from build123d import *

# Parameters (mm, degrees)
EXTRUDE_1_DEPTH = 2
SKETCH_2_R      = 4.1
EXTRUDE_2_DEPTH = 15


with BuildPart() as part:
    # 草图1 → 凸台-拉伸1 (new body)
    with BuildSketch(Plane.XY):
        Polygon((-12.668616293, 22.288540635), (-0.168616293, 22.288540635), (-0.168616293, 19.288540635), (14.831383707, 19.288540635), (14.831383707, 22.288540635), (27.331383707, 22.288540635), (27.331383707, -2.711459365), (-12.668616293, -2.711459365), align=None)
        with BuildLine():
            Line((-7.668616293, 0.038540635), (22.331383707, 0.038540635))
            ThreePointArc((22.331383707, 0.038540635), (23.081383707, -0.711459365), (22.331383707, -1.461459365))
            Line((22.331383707, -1.461459365), (-7.668616293, -1.461459365))
            ThreePointArc((-7.668616293, -1.461459365), (-8.418616293, -0.711459365), (-7.668616293, 0.038540635))
        make_face(mode=Mode.SUBTRACT)
    extrude(amount=EXTRUDE_1_DEPTH)

    # 草图2 → 凸台-拉伸2 (add)
    with BuildSketch(Plane(origin=(0, 19.288540635, 0), x_dir=(1, 0, 0), z_dir=(0, 1, 0))):
        with BuildLine():
            Line((4.831383707, 2.381058819), (4.831383707, 0))
            Line((4.831383707, 0), (9.831383707, 0))
            Line((9.831383707, 0), (9.831383707, 2.399323324))
            ThreePointArc((9.831383707, 2.399323324), (7.288775956, 14.054276854), (4.831383707, 2.381058819))
        make_face()
        with Locations((7.311058504, 7.954317551)):
            Circle(SKETCH_2_R, mode=Mode.SUBTRACT)
    extrude(amount=-EXTRUDE_2_DEPTH)


solid = part.part
CAD build for the part. Positions are in the model's coordinates, mm. A direction names the side the tool comes from. Round coordinates to 2 decimals unless told otherwise and drop trailing zeros. Write each loop counter-clockwise with the first axis right and the second up, starting at its lowest first coordinate (ties: lowest second). Pieces come first, ordered by that corner, then holes. Notation, with made-up numbers: M 41,-18.75 L 61,-18.75 A31 cw 61,20.25 Z; hole C 78,-20 d5. An arc over 180 degrees is marked long. Use a Markdown table: item, result. Add a question column.
1. Pull direction Z, two halves, no side cores. Call faces 1 (the face through (3, 4.289, -7)), 2 (the face through (6.78, 11.89, -12.02)), 3 (the face through (8, 10, 2)): released by +Z, released by -Z, zero draft, split by the parting line, or undercut.
2. Drill centre lines: probe 1 along Z at (x, y) = (-6, 19.25); probe 2 along Y at (x, z) = (9.5, -1.75); probe 3 along Y at (x, z) = (-6, 1). Where is each one in solid material? Low to high.
3. Flat gauge pins, fed straight in: P1, Ø4.5, axis at x = 8.5, z = -5, coming from the +Y side; P2, Ø1.9, axis at y = 10.5, z = -1, coming from the +X side; P3, Ø0.7, axis at y = 14, z = -1, coming from the -X side. Where does each tip first touch, or does it go through?
4. Slice it at B-B on z = -5.75. Give the cut face in (x, y), then the cut area to 3 significant figures.
5. Slice it at D-D on x = 6. Give the cut face in (y, z).
6. Slice it at A-A on x = 14. Give the cut face in (y, z).
7. 3-axis set-ups, long thin cutter, end or side, ignore diameter. For faces 4 (the face through (-8.42, -0.73, 0.99)), 5 (the face through (-0.169, 21, 1)), 6 (the face through (4.831, 12, -1)), 7 (the face through (8, -2.711, 1)), 8 (the face through (9.831, 12, -1)): which of +Z, -Z, +X, -X, +Y, -Y reach the whole face in a straight line?
8. Slice it at C-C on y = 10.5. Give the cut face in (x, z), then the cut area to 3 significant figures.
Reply:
| question | item | result |
|---|---|---|
| 1 | face 1 | zero draft |
| 1 | face 2 | undercut |
| 1 | face 3 | released by +Z |
| 2 | probe 1 | z = 0 to 2 |
| 2 | probe 2 | y = 4.29 to 19.29 |
| 2 | probe 3 | y = -2.71 to -1.46, 0.04 to 22.29 |
| 3 | P1 | stops at y = 19.29 |
| 3 | P2 | stops at x = 9.83 |
| 3 | P3 | stops at x = 4.83 |
| 4 | outline | M 1.62,4.29 L 3.85,4.29 L 3.85,19.29 L 1.62,19.29 Z; M 10.77,4.29 L 13,4.29 L 13,19.29 L 10.77,19.29 Z |
| 4 | area | 66.9 mm^2 |
| 5 | outline | M -2.71,0 L -1.46,0 L -1.46,2 L -2.71,2 Z; M 0.04,0 L 4.29,0 L 4.29,-4.07 L 19.29,-4.07 L 19.29,2 L 0.04,2 Z; M 4.29,-13.91 L 19.29,-13.91 L 19.29,-11.84 L 4.29,-11.84 Z |
| 6 | outline | M -2.71,0 L -1.46,0 L -1.46,2 L -2.71,2 Z; M 0.04,0 L 19.29,0 L 19.29,2 L 0.04,2 Z |
| 7 | face 4 | +Z, -Z |
| 7 | face 5 | +Z, -Z, +Y |
| 7 | face 6 | -X, +Y, -Y |
| 7 | face 7 | +Z, -Z, +X, -X, -Y |
| 7 | face 8 | +X, +Y, -Y |
| 8 | outline | M -12.67,0 L 4.83,0 L 4.83,-2.38 A6.1 ccw long 9.83,-2.4 L 9.83,0 L 27.33,0 L 27.33,2 L -12.67,2 Z; hole C 7.31,-7.95 d8.2 |
| 8 | area | 154 mm^2 |
